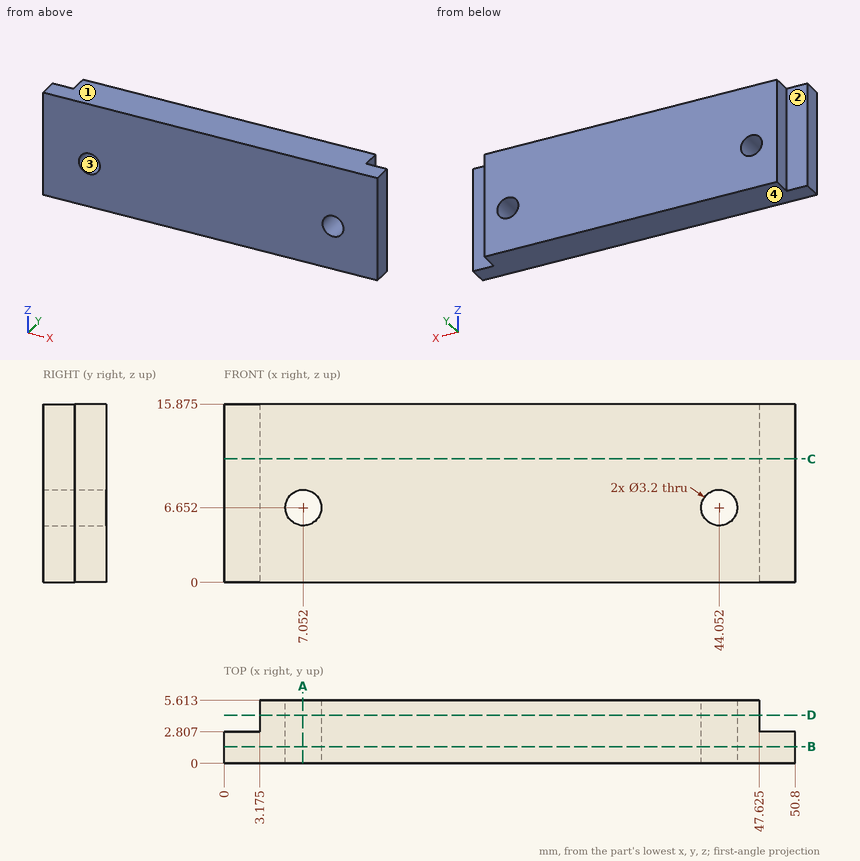
Drawing for the job (mm, zero at the part's lowest x, y, z). A direction names the side the tool comes from. Round coordinates to 2 decimals unless told otherwise and drop trailing zeros. Loops run counter-clockwise (first coordinate to the right, second up) from the corner with the lowest first, then second, coordinate; pieces in that order, holes last. Notation, with made-up numbers: (73.5, 25) -> (121.5, 25) arc R25 ccw to (121.5, 41) -> close; hole circle Ø10 at (51.5, 65.25). An arc over 180 degrees is marked (long way). Answer as CSV lines item,"result". Start each with the question number.
1) Slice it at D-D (y = 4.3). List the corners of the cut face in (x, z) (1 decimal).
2) Pin check, flat tips, straight feed: P1, Ø3.5, axis at x = 50, z = 8, coming from the +Y side; P2, Ø1.4, axis at y = 4, z = 12, coming from the -X side (3 decimals); P3, Ø1.4, axis at y = 4, z = 11, coming from the +X side (3 decimals). Stop position of each tip, or through.
3) Probe line 1 along X through (y, z) = (4.1, 7.5) (1 decimal); line 2 along X through (y, z) = (4.1, 8.5) (1 decimal); line 3 along X through (y, z) = (0.5, 5.25) (1 decimal). List the from-to ranges inside material, lowest first.
4) Tool access for the marked faces 1 and 2: list every direction of +Z, -Z, +X, -X, +Y, -Y with a clear straight run to the whole face (end or side of a thin tool).
5) Slice it at C-C (z = 11). List the corners of the cut face in (x, y) (1 decimal), plus the area to 3 significant figures.
6) Slice it at B-B (y = 1.5). List the corners of the cut face in (x, z) (1 decimal), plus the area to 3 significant figures.
7) Slice it at A-A (x = 7). List the corners of the cut face in (y, z) (1 decimal).
8) Mould opens along X. For the marked faces 3 and 4 say: +X half, -X half, draft (parallel to the pull), parting line (faces both ways), or undercut.
Filled in:
1,outline,"(3.2, 0) -> (47.6, 0) -> (47.6, 15.9) -> (3.2, 15.9) -> close; hole circle Ø3.2 at (7.1, 6.7); hole circle Ø3.2 at (44.1, 6.7)"
2,P1,"stops at y = 2.81"
2,P2,"stops at x = 3.175"
2,P3,"stops at x = 47.625"
3,line 1,"x = 3.2 to 5.7, 8.4 to 42.7, 45.4 to 47.6"
3,line 2,"x = 3.2 to 47.6"
3,line 3,"x = 0 to 6.3, 7.8 to 43.3, 44.8 to 50.8"
4,face 1,"+Z, +X, -X, +Y, -Y"
4,face 2,"+Z, -Z, -X, +Y"
5,outline,"(0, 0) -> (50.8, 0) -> (50.8, 2.8) -> (47.6, 2.8) -> (47.6, 5.6) -> (3.2, 5.6) -> (3.2, 2.8) -> (0, 2.8) -> close"
5,area,"267 mm2"
6,outline,"(0, 0) -> (50.8, 0) -> (50.8, 15.9) -> (0, 15.9) -> close; hole circle Ø3.2 at (7.1, 6.7); hole circle Ø3.2 at (44.1, 6.7)"
6,area,"790 mm2"
7,outline,"(0, 0) -> (5.6, 0) -> (5.6, 5.1) -> (0, 5.1) -> close; (0, 8.3) -> (5.6, 8.3) -> (5.6, 15.9) -> (0, 15.9) -> close"
8,face 3,"undercut"
8,face 4,"draft"
